The listing builds one solid part. Answer for the finished solid, in the listing's coordinates (mm). A direction names the side the tool comes from. Coordinates: 2 decimals unless noted, no trailing zeros. Loops run counter-clockwise (first coordinate to the right, second up) from the corner with the lowest first, then second, coordinate; pieces in that order, holes last. Notation, with made-up numbers: M -15,-3 L 36,-3 A29 ccw 36,28 Z; hole C 57,8.5 d9. An arc over 180 degrees is marked long. Answer as CSV lines item,"result". Start each with the question number.
```python
from build123d import *

# Parameters (mm, degrees)
CHAMFER_1_SIZE              = 1
CUT_EXTRUDE_START           = -22
SKETCH_2_OUTSIDE_W          = 62.6
SKETCH_2_OUTSIDE_H          = 62.6
SKETCH_2_OUTSIDE_R          = 13
CUT_EXTRUDE_1_DEPTH         = 2
CUT_EXTRUDE_START_2         = -14
CUT_EXTRUDE_2_DEPTH         = 14
CHAMFER_2_SIZE              = 2
CUT_EXTRUDE_START_3         = 3.5
CUT_EXTRUDE_3_DEPTH         = 123.809144562
HOLE_WIZARD_14_0_14_1_D     = 14
HOLE_WIZARD_14_0_14_1_DEPTH = 16
HOLE_WIZARD_14_0_14_1_TIP   = 4.206024333
CHAMFER_3_SIZE              = 1


# Read off the part's stored shape, not the designer's step: M30 机械螺纹 螺柱1, 切除-拉伸2
with BuildPart() as part:
    # 草图1 → 旋转1 (revolve)
    with BuildSketch(Plane.XY):
        Polygon((0, 0), (0, 6), (2.5, 6), (2.5, 5.5), (3.5, 5.5), (3.5, 6), (18.5, 6), (18.5, 5.5), (19.5, 5.5), (19.5, 7.5), (64, 7.5), (64, 6.5), (66, 6.5), (66, 17), (124, 17), (124, 0), align=None)
    revolve(axis=Axis((124, 0, 0), (-1, 0, 0)))

    # 倒角1
    chamfer_1_edges = [part.edges().sort_by_distance(p)[0] for p in [
        (66, -17, 0),
        (0, -6, 0),
    ]]
    chamfer(chamfer_1_edges, length=CHAMFER_1_SIZE)

    # 草图2 outside → 切除-拉伸1 (cut)
    with BuildSketch(Plane(origin=(124, 0, 0), x_dir=(0, 0, -1), z_dir=(1, 0, 0)).offset(CUT_EXTRUDE_START)):
        Rectangle(SKETCH_2_OUTSIDE_W, SKETCH_2_OUTSIDE_H)
        with Locations(Location((0, 0, 0), (0, 0, 90))):
            Circle(SKETCH_2_OUTSIDE_R, mode=Mode.SUBTRACT)
    extrude(amount=CUT_EXTRUDE_1_DEPTH, mode=Mode.SUBTRACT)

    # M30 机械螺纹 螺柱1 outline → M30 机械螺纹 螺柱1 (revolve, cut)
    with BuildSketch(Plane.YX):
        Polygon((17, 124), (13.1055, 124), (15, 122.1055), (15, 104), (17, 104), align=None)
    revolve(axis=Axis((0, 0, 0), (1, 0, 0)), mode=Mode.SUBTRACT)

    # 切除-拉伸2 outline → 切除-拉伸2 (cut)
    with BuildSketch(Plane(origin=(102, 0, 0), x_dir=(0, 0, -1), z_dir=(1, 0, 0)).offset(CUT_EXTRUDE_START_2)):
        with BuildLine():
            Line((-8, 15), (8, 15))
            ThreePointArc((8, 15), (0, 17), (-8, 15))
        make_face()
        with BuildLine():
            Line((8, -15), (-8, -15))
            ThreePointArc((-8, -15), (0, -17), (8, -15))
        make_face()
    extrude(amount=CUT_EXTRUDE_2_DEPTH, mode=Mode.SUBTRACT)

    # 倒角2
    chamfer_2_edges = [part.edges().sort_by_distance(p)[0] for p in [
        (88, -15, 0),
        (88, 15, 0),
    ]]
    chamfer(chamfer_2_edges, length=CHAMFER_2_SIZE - 0.0001)  # a hair under: the kernel refuses the full size

    # 草图5 → 切除-拉伸3 (cut, through all)
    with BuildSketch(Plane(origin=(0, 0, 0), x_dir=(1, 0, 0), z_dir=(0, 1, 0)).offset(CUT_EXTRUDE_START_3)):
        with BuildLine():
            Line((15.5, -2), (7.5, -2))
            ThreePointArc((7.5, -2), (5.5, 0), (7.5, 2))
            Line((7.5, 2), (15.5, 2))
            ThreePointArc((15.5, 2), (17.5, 0), (15.5, -2))
        make_face()
    extrude(amount=CUT_EXTRUDE_3_DEPTH, mode=Mode.SUBTRACT)

    # 草图6 → 切除-旋转1 (revolve, cut)
    with BuildSketch(Plane.XY):
        Polygon((92, 0), (92, 9.5), (97, 9.5), (97, 9), (103, 9), (103, 9.5), (108, 9.5), (108, 8.680110408), (124, 11), (124, 0), align=None)
    revolve(axis=Axis((124, 0, 0), (-1, 0, 0)), mode=Mode.SUBTRACT)

    # Ø14.0 (14) 直径孔1
    with Locations(Plane(origin=(92, 0, 0), x_dir=(0, 0, -1), z_dir=(1, 0, 0))):
        with Locations((0, 0)):
            Hole(HOLE_WIZARD_14_0_14_1_D / 2, depth=HOLE_WIZARD_14_0_14_1_DEPTH)
            with Locations((0, 0, -(HOLE_WIZARD_14_0_14_1_DEPTH + HOLE_WIZARD_14_0_14_1_TIP / 2))):  # 118° drill point
                Cone(0, HOLE_WIZARD_14_0_14_1_D / 2, HOLE_WIZARD_14_0_14_1_TIP, mode=Mode.SUBTRACT)

    # 倒角3
    chamfer_3_edges = [part.edges().sort_by_distance(p)[0] for p in [
        (92, 0, -7),
    ]]
    chamfer(chamfer_3_edges, length=CHAMFER_3_SIZE)


solid = part.part
```
Item 1: Consider line 1 (Z direction, x = 94.95, y = 0); line 2 (Y direction, x = 95, z = 0); line 3 (Z direction, x = 101.1, y = 0). Determine where each line is inside the solid, lowest interval first.
Item 2: For a pull along Z with two mould halves and no side action, classify faces 1 (the face through (100.042, -1.172, -8.923)), 2 (the face through (18.5, 3, 5)), 3 (the face through (19.01, -1.19, 5.37)), 4 (the face through (12, 3.5, 0)) as pulls with the +Z half, pulls with the -Z half, needs draft (parallel to the pull), parting line crosses it, or undercut.
Item 3: Each of these flat-tipped pins is pushed along its axis until it touches: P1, Ø9.5, axis at y = 3, z = 0.5, coming from the +X side; P2, Ø1.5, axis at x = 30.5, z = -6, coming from the +Y side; P3, Ø6, axis at x = 16, z = -1, coming from the -Y side. Where does it stop, or does it pass through?
Item 4: For faces 5 (the face through (83.395, -2.681, 6.466)), 6 (the face through (103, 6, 7)), 7 (the face through (11, 5, -2)), 8 (the face through (2, -6, 0)), determine the directions among +Z, -Z, +X, -X, +Y, -Y from which every point of the face is accessible in a straight line to the end or side of a thin tool.
Item 5: Section B-B on x = 115 is taken. Determine the outline of the cut face in (y, z), then the cut area to 3 significant figures.
Item 6: Section A-A on x = 54 is taken. Determine the outline of the cut face in (y, z).
Results are:
1,line 1,"-17 to -9.5, 9.5 to 17"
1,line 2,"-15 to -9.5, 9.5 to 15"
1,line 3,"-17 to -9, 9 to 17"
2,face 1,"undercut"
2,face 2,"needs draft"
2,face 3,"parting line crosses it"
2,face 4,"undercut"
3,P1,"x = 91.79"
3,P2,"y = 5.36"
3,P3,"y = -6"
4,face 5,"+X"
4,face 6,"none"
4,face 7,"+Y"
4,face 8,"-X"
5,outline,"C 0,0 d30; hole C 0,0 d19.39"
5,area,"412 mm²"
6,outline,"C 0,0 d15"
